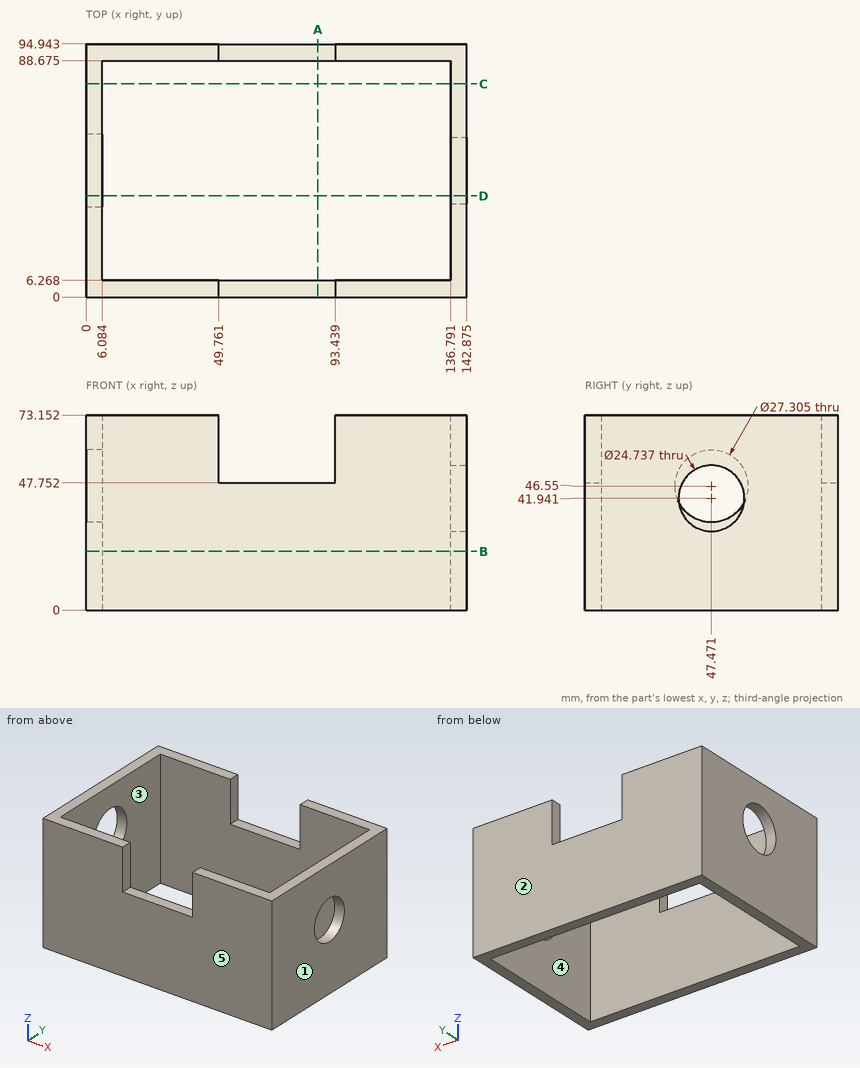
Drawing for the job (mm, zero at the part's lowest x, y, z). A direction names the side the tool comes from. Give positions to 0.01 mm unless a question says otherwise; leave off trailing zeros. Order: outer loops, then holes, each group sorted by start corner. A loop starts at its lowest first (then second) coordinate and runs counter-clockwise, first axis right, second up. Notation, with made-up numbers: M 73,75 L 132,75 A10 cw 132,94 Z; hole C -10.5,-13.75 d8. An arc over 180 degrees is marked long. Use a Markdown table: item, result. Add a question column.
(1) Saw through at C-C, the plane y = 80. Give the cut face in (x, z) (1 decimal).
(2) Saw through at B-B, the plane z = 22. Give the cut face in (x, y) (1 decimal), and give its area (3 significant figures).
(3) Saw through at D-D, the plane y = 38. Give the cut face in (x, z) (1 decimal).
(4) 3-axis set-ups, long thin cutter, end or side, ignore diameter. For the marked faces 4 and 5: which of +Z, -Z, +X, -X, +Y, -Y reach the whole face in a straight line?
(5) Saw through at A-A, the plane x = 87. Give the cut face in (y, z) (1 decimal).
(6) Drop a flat-ended pin along its axis: P1, Ø5, axis at x = 68, y = 3, coming from the +Z side. Give the stop position or say it passes through.
(7) Mould opens along Y. For the marked faces 1, 2 and 3 say: +Y half, -Y half, draft (parallel to the pull), parting line (faces both ways), or undercut.
(8) Probe line 1 along X through (y, z) = (81, 3) (1 decimal); line 2 along Y through (x, z) = (136.5, 24) (1 decimal). List the from-to ranges inside material, lowest first. Write a range as [from, to].
Answer key:
| question | item | result |
|---|---|---|
| 1 | outline | M 0,0 L 6.1,0 L 6.1,73.2 L 0,73.2 Z; M 136.8,0 L 142.9,0 L 142.9,73.2 L 136.8,73.2 Z |
| 2 | outline | M 0,0 L 142.9,0 L 142.9,94.9 L 0,94.9 Z; hole M 6.1,6.3 L 136.8,6.3 L 136.8,88.7 L 6.1,88.7 Z |
| 2 | area | 2,790 mm^2 |
| 3 | outline | M 0,0 L 6.1,0 L 6.1,36.7 L 0,36.7 Z; M 0,56.4 L 6.1,56.4 L 6.1,73.2 L 0,73.2 Z; M 136.8,0 L 142.9,0 L 142.9,34 L 136.8,34 Z; M 136.8,49.9 L 142.9,49.9 L 142.9,73.2 L 136.8,73.2 Z |
| 4 | face 4 | +Z, -Z |
| 4 | face 5 | +Z, -Z, +X, -X, -Y |
| 5 | outline | M 0,0 L 6.3,0 L 6.3,47.8 L 0,47.8 Z; M 88.7,0 L 94.9,0 L 94.9,47.8 L 88.7,47.8 Z |
| 6 | P1 | z = 47.75 |
| 7 | face 1 | draft |
| 7 | face 2 | +Y half |
| 7 | face 3 | undercut |
| 8 | line 1 | [0, 6.1], [136.8, 142.9] |
| 8 | line 2 | [0, 6.3], [88.7, 94.9] |
